Geometry check sheet. Reference: the model listing, model coordinates, mm. Face numbers are marked on the shaded views. A direction names the side the tool comes from. Give positions to 0.01 mm unless a question says otherwise; leave off trailing zeros. Write each loop counter-clockwise with the first axis right and the second up, starting at its lowest first coordinate (ties: lowest second). Pieces come first, ordered by that corner, then holes. Notation, with made-up numbers: M 3.25,52 L 51.25,52 A28 cw 51.25,79 Z; hole C -21,67 d10. An arc over 180 degrees is marked long. One line per item, written item: value. Start each with the question number.
1. Release check for a two-part mould opening along Y. For the marked faces 1, 2 and 3 record: pulls with the +Y half, pulls with the -Y half, needs draft (parallel to the pull), parting line crosses it, or undercut.
2. Gauge pin test, flat ends, axial feed: pin 1 (8 mm diameter, centred on x = -12.5, y = -1.5, fed in from -Z); pin 2 (2 mm diameter, centred on x = 11.5, z = 5.5, fed in from -Y); pin 3 (1.5 mm diameter, centred on x = -4, z = 11, fed in from -Y); pin 4 (3.5 mm diameter, centred on x = -4, z = 10, fed in from +Y). Record the tip position at first contact, or that the pin passes through.
3. Scan lines: line 1 (X direction, y = -3.5, z = 9); line 2 (Y direction, x = 0, z = 3.2). Record each from-to range of solid material in increasing order.
4. Tool access check on the marked faces 4, 5 and 6. Record the directions out of +Z, -Z, +X, -X, +Y, -Y that give a thin tool (end or side, any length) a straight path to the whole face; none if there is none.
5. Cross-section at A-A on x = 0. Record the cut outline in (y, z).
6. Cross-section at B-B on z = 4. Record the cut outline in (x, y), then the cut area to 3 significant figures.
from build123d import *

# Parameters (mm, degrees)
CROQUIS1_R              = 20
SALIENTE_EXTRUIR1_DEPTH = 5
CROQUIS2_R              = 2.5
CORTAR_EXTRUIR1_DEPTH   = 5
CROQUIS3_W              = 5
CROQUIS3_H              = 15
SALIENTE_EXTRUIR3_DEPTH = 15
CROQUIS4_R              = 2.5
CORTAR_EXTRUIR2_DEPTH   = 5
FILLET1_R               = 2
FILLET2_R               = 2.5


with BuildPart() as part:
    # Croquis1 → Saliente-Extruir1 (new body)
    with BuildSketch(Plane.XY):
        Circle(CROQUIS1_R)
    extrude(amount=SALIENTE_EXTRUIR1_DEPTH)

    # Croquis2 → Cortar-Extruir1 (cut)
    with BuildSketch(Plane.XY.offset(5)):
        Circle(CROQUIS2_R)
    extrude(amount=-CORTAR_EXTRUIR1_DEPTH, mode=Mode.SUBTRACT)

    # Croquis3 → Saliente-Extruir3 (add)
    with BuildSketch(Plane.XY.offset(5)):
        with Locations((5, 0)):
            Rectangle(CROQUIS3_W, CROQUIS3_H)
    extrude(amount=SALIENTE_EXTRUIR3_DEPTH)

    # Croquis4 → Cortar-Extruir2 (cut)
    with BuildSketch(Plane(origin=(7.5, 0, 0), x_dir=(0, 0, -1), z_dir=(1, 0, 0))):
        with BuildLine():
            ThreePointArc((-12.5, -7.5), (-17.803300859, -5.303300859), (-20, 0))
            Line((-20, 0), (-20, -7.5))
            Line((-20, -7.5), (-12.5, -7.5))
        make_face()
        with BuildLine():
            ThreePointArc((-20, 0), (-17.803300859, 5.303300859), (-12.5, 7.5))
            Line((-12.5, 7.5), (-20, 7.5))
            Line((-20, 7.5), (-20, 0))
        make_face()
        with Locations((-12.5, 0)):
            Circle(CROQUIS4_R)
    extrude(amount=-CORTAR_EXTRUIR2_DEPTH, mode=Mode.SUBTRACT)

    # Simetría1: part across plane


with BuildPart() as part_1:
    add(part.part)
    add(part.part.mirror(Plane(origin=(0, 0, 0), x_dir=(0, 0, 1), z_dir=(1, 0, 0))))

    # Fillet1
    fillet1_edges = [part_1.edges().sort_by_distance(p)[0] for p in [
        (5, -7.5, 5),
        (7.5, 0, 5),
        (5, 7.5, 5),
        (7.5, -7.5, 8.75),
        (7.5, 0, 20),
        (7.5, 7.5, 8.75),
        (-5, -7.5, 5),
        (-7.5, 0, 5),
        (-5, 7.5, 5),
        (-7.5, 7.5, 8.75),
        (-7.5, -7.5, 8.75),
        (-7.5, 0, 20),
    ]]
    fillet(fillet1_edges, radius=FILLET1_R)

    # Fillet2
    fillet2_edges = [part_1.edges().sort_by_distance(p)[0] for p in [
        (-20, 0, 5),
    ]]
    fillet(fillet2_edges, radius=FILLET2_R)


solid = part_1.part
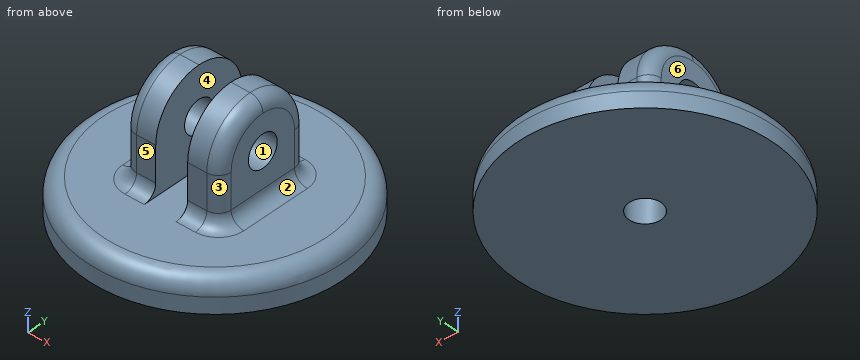
Report:
1. face 1: undercut
1. face 2: needs draft
1. face 3: pulls with the -Y half
2. pin 1: stops at z = 0
2. pin 2: stops at y = -15.28
2. pin 3: stops at y = -7.5
2. pin 4: stops at y = 7.5
3. line 1: x = -7.5 to -2.5, 2.5 to 7.5
3. line 2: y = -19.9 to -2.5, 2.5 to 19.9
4. face 4: +Z, +Y, -Y
4. face 5: +Z, +X, -X, -Y
4. face 6: +Z, -X, +Y, -Y
5. outline: M -20,0 L -2.5,0 L -2.5,5 L -17.5,5 A2.5 ccw -20,2.5 Z; M 2.5,0 L 20,0 L 20,2.5 A2.5 ccw 17.5,5 L 2.5,5 Z
6. outline: C 0,0 d39; hole C 0,0 d5
6. area: 1,170 mm^2
